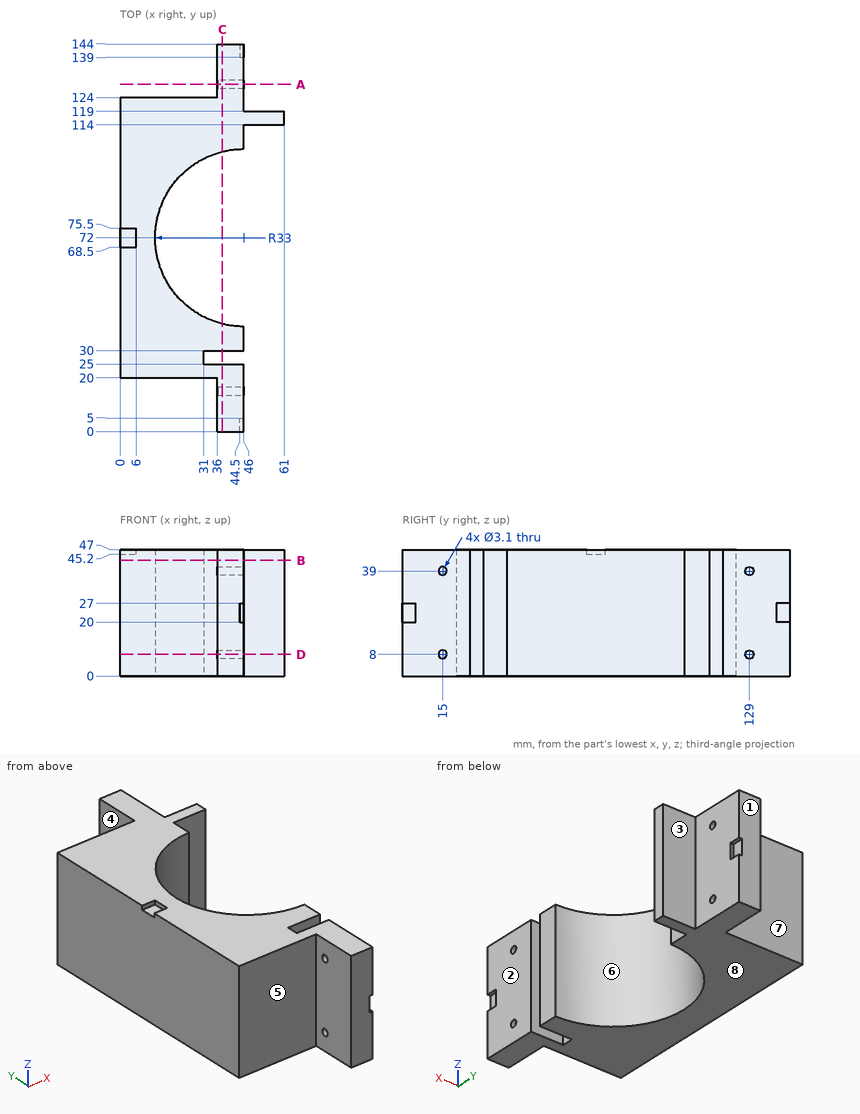
The figure shows three views and two pictorial views of one solid part (mm, origin at its lowest corner). Answer the questions. A direction names the side the tool comes from. Give positions to 0.01 mm unless a question says otherwise; leave off trailing zeros. Write each loop counter-clockwise with the first axis right and the second up, starting at its lowest first coordinate (ties: lowest second). Pieces come first, ordered by that corner, then holes. Notation, with made-up numbers: M -25.75,8 L -8.75,8 A28 ccw -8.75,31 Z; hole C 46,-24 d7. An arc over 180 degrees is marked long. One line per item, written item: value. Start each with the question number.
(1) Flat-ended cylindrical pins translate along their axes: pin 1 Ø1.5 at (y, z) = (141.5, 22) entering from +X; pin 2 Ø8 at (x, z) = (27, 8.5) entering from +Y; pin 3 Ø3 at (x, y) = (47.5, 41.5) entering from +Z; pin 4 Ø1.5 at (y, z) = (19.5, 15.5) entering from +X. Find the tip coordinate at first contact, or state that the pin passes through.
(2) Find section B-B (z = 43). Determine the outline of the cut face in (x, y), plus the area to 3 significant figures.
(3) Determine the mould class of the marked faces 6, 7 and 8 for opening direction Y: pulls with the +Y half, pulls with the -Y half, needs draft (parallel to the pull), parting line crosses it, or undercut.
(4) Find section C-C (x = 38). Determine the outline of the cut face in (y, z), plus the area to 3 significant figures.
(5) Find section D-D (z = 8). Determine the outline of the cut face in (x, y).
(6) Find the intervals of material crossed by line 1 (Z direction, x = 41, y = 15); line 2 (Y direction, x = 39, z = 8); line 3 (Y direction, x = 32.5, z = 44), in increasing order.
(7) A tool of negligible diameter and unlimited length cuts with its end or side. For the marked faces 1, 2, 3, 4 and 5, from which of +Z, -Z, +X, -X, +Y, -Y can it reach the whole face along a straight path? Write none if from no direction.
(8) Find section A-A (y = 129). Determine the outline of the cut face in (x, z).
Results below:
1. pin 1: stops at x = 44.5
1. pin 2: stops at y = 124
1. pin 3: passes through
1. pin 4: stops at x = 46
2. outline: M 0,20 L 36,20 L 36,0 L 46,0 L 46,25 L 31,25 L 31,30 L 46,30 L 46,39 A33 cw 46,105 L 46,114 L 61,114 L 61,119 L 46,119 L 46,144 L 36,144 L 36,124 L 0,124 Z
2. area: 3,470 mm^2
3. face 6: undercut
3. face 7: pulls with the +Y half
3. face 8: needs draft
4. outline: M 0,0 L 25,0 L 25,47 L 0,47 Z; M 30,0 L 39.98,0 L 39.98,47 L 30,47 Z; M 104.02,0 L 144,0 L 144,47 L 104.02,47 Z; hole C 15,8 d3.1; hole C 15,39 d3.1; hole C 129,8 d3.1; hole C 129,39 d3.1
4. area: 3,490 mm^2
5. outline: M 0,20 L 36,20 L 36,16.55 L 46,16.55 L 46,25 L 31,25 L 31,30 L 46,30 L 46,39 A33 cw 46,105 L 46,114 L 61,114 L 61,119 L 46,119 L 46,127.45 L 36,127.45 L 36,124 L 0,124 Z; M 36,0 L 46,0 L 46,13.45 L 36,13.45 Z; M 36,130.55 L 46,130.55 L 46,144 L 36,144 Z
6. line 1: z = 0 to 6.45, 9.55 to 37.45, 40.55 to 47
6. line 2: y = 0 to 13.45, 16.55 to 25, 30 to 39.75, 104.25 to 127.45, 130.55 to 144
6. line 3: y = 20 to 25, 30 to 41.89, 102.11 to 124
7. face 1: +Z, -Z, +X, -X, +Y
7. face 2: +Z, -Z, +X, -Y
7. face 3: +Z, -Z, +X, +Y
7. face 4: +Z, -Z, -X, +Y
7. face 5: +Z, -Z, -X, -Y
8. outline: M 36,0 L 46,0 L 46,6.45 L 36,6.45 Z; M 36,9.55 L 46,9.55 L 46,37.45 L 36,37.45 Z; M 36,40.55 L 46,40.55 L 46,47 L 36,47 Z
